Geometry: final body of the model. Coordinates: model frame, mm. Face numbers are marked on the shaded views. A direction names the side the tool comes from. Give positions to 0.01 mm unless a question says otherwise; leave off trailing zeros. Write each loop counter-clockwise with the first axis right and the second up, starting at its lowest first coordinate (ties: lowest second). Pieces come first, ordered by that corner, then holes.
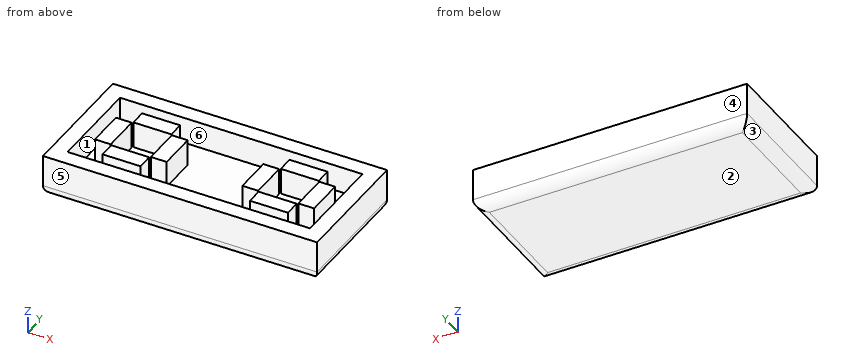
from build123d import *

# Parameters (mm, degrees)
SKETCH_W      = 12.985
SKETCH_H      = 12
PAD_DEPTH     = 1.5
PAD001_DEPTH  = 2.5
SKETCH002_W   = 3.6
SKETCH002_H   = 1.5
SKETCH002_W_2 = 1.5
SKETCH002_H_2 = 3.6
PAD002_DEPTH  = 4
FILLET_R      = 1


with BuildPart() as part:
    # Sketch → Pad (new body)
    with BuildSketch(Plane.XY):
        with Locations((-6.4925, 0)):
            Rectangle(SKETCH_W, SKETCH_H)
    pad = extrude(amount=PAD_DEPTH)

    # Sketch001 → Pad001 (join)
    with BuildSketch(Plane.XY.offset(1.5)):
        Polygon((-12.985, 6), (0, 6), (0, 4.5), (-11.485, 4.5), (-11.485, -4.5), (0, -4.5), (0, -6), (-12.985, -6), align=None)
    pad001 = extrude(amount=PAD001_DEPTH)

    # Sketch002 → Pad002 (join)
    with BuildSketch(Plane.XY):
        with Locations((-6.985, 2.65)):
            Rectangle(SKETCH002_W, SKETCH002_H)
        with Locations((-6.985, -2.65)):
            Rectangle(SKETCH002_W, SKETCH002_H)
        with Locations((-9.635, 0)):
            Rectangle(SKETCH002_W_2, SKETCH002_H_2)
        with Locations((-4.335, 0)):
            Rectangle(SKETCH002_W_2, SKETCH002_H_2)
    pad002 = extrude(amount=PAD002_DEPTH)

    # Mirrored: Pad across Sketch V_Axis
    add(pad.mirror(Plane(origin=(0, 0, 0), x_dir=(0, 0, 1), z_dir=(1, 0, 0))))

    # Mirrored001: Pad002 across Sketch002 V_Axis
    add(pad002.mirror(Plane(origin=(0, 0, 0), x_dir=(0, 0, 1), z_dir=(1, 0, 0))))

    # Mirrored002: Pad001 across Sketch001 V_Axis
    add(pad001.mirror(Plane(origin=(0, 0, 1.5), x_dir=(0, 0, 1), z_dir=(1, 0, 0))))

    # Fillet
    fillet_edges = [part.edges().sort_by_distance(p)[0] for p in [
        (12.985, 0, 0),
        (0, -6, 0),
        (-12.985, 0, 0),
        (0, 6, 0),
    ]]
    fillet(fillet_edges, radius=FILLET_R)


solid = part.part
Q1. Access query for the marked faces 1 and 2. Directions: +Z, -Z, +X, -X, +Y, -Y. A direction counts if a zero-diameter tool reaches every point of the face in a straight line with its end or side. Return the directions, or none.
Filled sheet:
face 1: +Z
face 2: -Z, +X, -X, +Y, -Y
Q2. Pull-direction query (Y, two-part tool) for the marked faces 3, 4, 5 and 6; classes: released by +Y, released by -Y, zero draft, split by the parting line, or undercut.
Filled sheet:
face 3: zero draft
face 4: released by +Y
face 5: released by -Y
face 6: undercut
Q3. Ray query, line 1 along Y through (x, z) = (-4.25, 1.9); line 2 along X through (y, z) = (-1.25, 2.3) (3 decimals); line 3 along Y through (x, z) = (-5.25, 3.55). Return the intervals inside material, ascending.
Filled sheet:
line 1: y = -6 to -4.5, -1.8 to 1.8, 4.5 to 6
line 2: x = -12.985 to -11.485, -10.385 to -8.885, -5.085 to -3.585, 3.585 to 5.085, 8.885 to 10.385, 11.485 to 12.985
line 3: y = -6 to -4.5, -3.4 to -1.9, 1.9 to 3.4, 4.5 to 6
Q4. Section B-B on x = 0. Output: boundary loops of the cut face in (y, z), plus the area to 3 significant figures.
Filled sheet:
outline: (-6, 1) arc R1 ccw to (-5, 0) - (5, 0) arc R1 ccw to (6, 1) - (6, 4) - (4.5, 4) - (4.5, 1.5) - (-4.5, 1.5) - (-4.5, 4) - (-6, 4) - close
area: 25.1 mm2
Q5. Section D-D on y = 1.5. Output: boundary loops of the cut face in (x, z) (3 decimals), plus the area to 3 significant figures.
Filled sheet:
outline: (-12.985, 1) arc R1 ccw to (-11.985, 0) - (11.985, 0) arc R1 ccw to (12.985, 1) - (12.985, 4) - (11.485, 4) - (11.485, 1.5) - (10.385, 1.5) - (10.385, 4) - (8.885, 4) - (8.885, 1.5) - (5.085, 1.5) - (5.085, 4) - (3.585, 4) - (3.585, 1.5) - (-3.585, 1.5) - (-3.585, 4) - (-5.085, 4) - (-5.085, 1.5) - (-8.885, 1.5) - (-8.885, 4) - (-10.385, 4) - (-10.385, 1.5) - (-11.485, 1.5) - (-11.485, 4) - (-12.985, 4) - close
area: 61.0 mm2
Q6. Section A-A on y = -4.25. Output: boundary loops of the cut face in (x, z) (3 decimals).
Filled sheet:
outline: (-12.985, 1) arc R1 ccw to (-11.985, 0) - (11.985, 0) arc R1 ccw to (12.985, 1) - (12.985, 4) - (11.485, 4) - (11.485, 1.5) - (-11.485, 1.5) - (-11.485, 4) - (-12.985, 4) - close
Q7. Section C-C on z = 1.9. Count the separate pieces of the cut face and the enclosed holes in it, plus the area to 3 significant figures.
Filled sheet:
separate pieces: 9
enclosed holes: 1
area: 148 mm2
